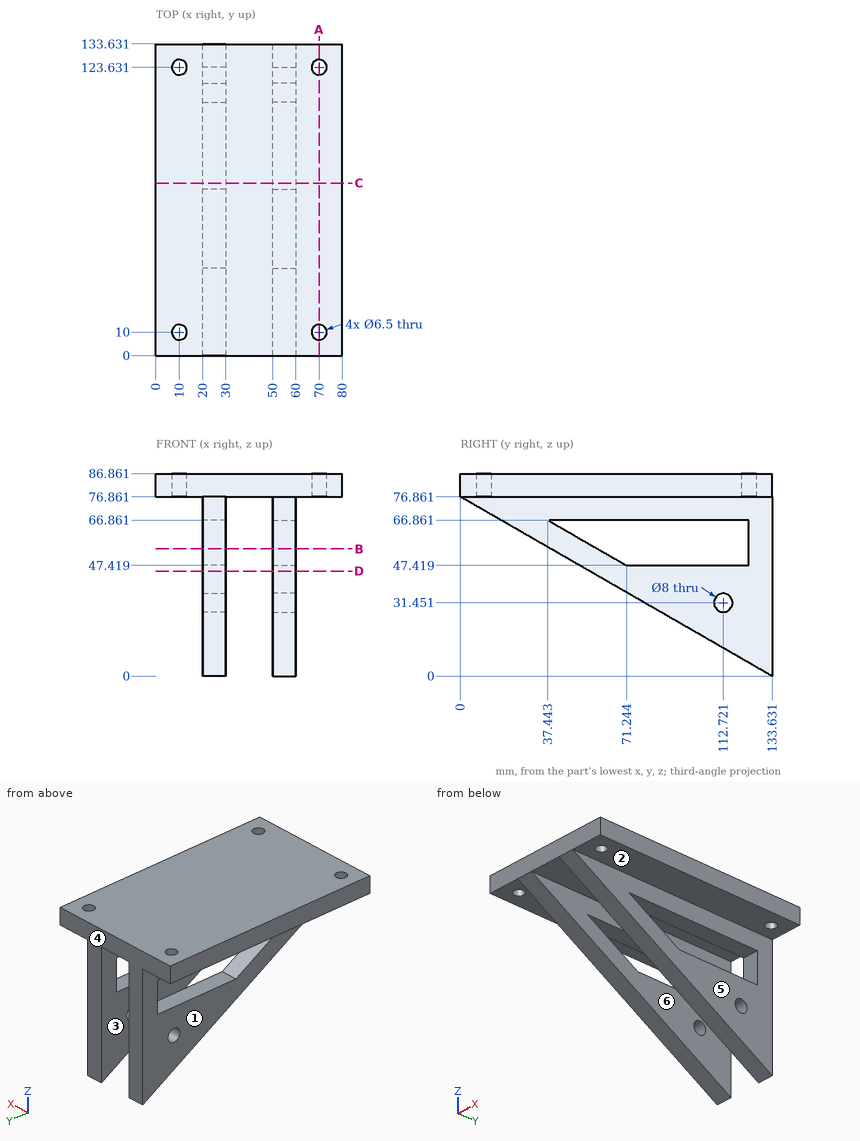
Study the drawing (mm; zero at the part's minimum x, y, z) and answer. A direction names the side the tool comes from. Give positions to 0.01 mm unless a question says otherwise; leave off trailing zeros. Order: outer loops, then holes, each group sorted by start corner. A loop starts at its lowest first (then second) coordinate and runs counter-clockwise, first axis right, second up. Notation, with made-up numbers: (7.25, 3) -> (11.25, 3) arc R25 cw to (11.25, 38) -> close; hole circle Ø4 at (75, 28). An arc over 180 degrees is marked (long way). Write item = value, one per line.
1. Given pin 1 (5 mm diameter, centred on x = 70, y = 10, fed in from +Z); pin 2 (3 mm diameter, centred on x = 38.5, y = 16.5, fed in from -Z); pin 3 (12 mm diameter, centred on y = 120, z = 25.5, fed in from -X); pin 4 (7.5 mm diameter, centred on x = 70, y = 123.63, fed in from +Z), each flat-ended and moving along its own axis, determine where each tip first touches the part or whether it passes through.
Numbers:
pin_1 = through
pin_2 = 76.86
pin_3 = 20
pin_4 = 86.86
2. The mould has two halves that part along X. Classify the marked faces 1, 2 and 3: +X half, -X half, draft (parallel to the pull), parting line (faces both ways), or undercut.
Numbers:
face_1 = -X half
face_2 = draft
face_3 = undercut
3. A cutting plane is placed at A-A, the plane x = 70. Write down the section's boundary in (y, z).
Numbers:
outline = (0, 76.86) -> (6.75, 76.86) -> (6.75, 86.86) -> (0, 86.86) -> close; (13.25, 76.86) -> (120.38, 76.86) -> (120.38, 86.86) -> (13.25, 86.86) -> close; (126.88, 76.86) -> (133.63, 76.86) -> (133.63, 86.86) -> (126.88, 86.86) -> close
4. For the marked faces 4, 5 and 6, determine the directions among +Z, -Z, +X, -X, +Y, -Y from which every point of the face is accessible in a straight line to the end or side of a thin tool.
Numbers:
face_4 = +Z, -Z, +X, -X, +Y
face_5 = -Z, +X, +Y, -Y
face_6 = -Z, +Y, -Y
5. A cutting plane is placed at D-D, the plane z = 45. Write down the section's boundary in (x, y).
Numbers:
outline = (20, 55.39) -> (30, 55.39) -> (30, 133.63) -> (20, 133.63) -> close; (50, 55.39) -> (60, 55.39) -> (60, 133.63) -> (50, 133.63) -> close
6. A cutting plane is placed at B-B, the plane z = 54.5. Write down the section's boundary in (x, y), and give its area (3 significant figures).
Numbers:
outline = (20, 38.88) -> (30, 38.88) -> (30, 58.93) -> (20, 58.93) -> close; (20, 123.63) -> (30, 123.63) -> (30, 133.63) -> (20, 133.63) -> close; (50, 38.88) -> (60, 38.88) -> (60, 58.93) -> (50, 58.93) -> close; (50, 123.63) -> (60, 123.63) -> (60, 133.63) -> (50, 133.63) -> close
area = 601 mm²
7. Straight lines are drawn through the part: line 1 along Y through (x, z) = (10, 84); line 2 along X through (y, z) = (37, 58.5); line 3 along Z through (x, y) = (66.5, 78). For each, find the intervals that lie inside material, in ascending order.
Numbers:
line_1 = 0 to 6.75, 13.25 to 120.38, 126.88 to 133.63
line_2 = 20 to 30, 50 to 60
line_3 = 76.86 to 86.86
8. A cutting plane is placed at C-C, the plane y = 74. Write down the section's boundary in (x, z).
Numbers:
outline = (0, 76.86) -> (20, 76.86) -> (20, 66.86) -> (30, 66.86) -> (30, 76.86) -> (50, 76.86) -> (50, 66.86) -> (60, 66.86) -> (60, 76.86) -> (80, 76.86) -> (80, 86.86) -> (0, 86.86) -> close; (20, 34.3) -> (30, 34.3) -> (30, 47.42) -> (20, 47.42) -> close; (50, 34.3) -> (60, 34.3) -> (60, 47.42) -> (50, 47.42) -> close
